```python
from build123d import *

# Parameters (mm, degrees)
F0_W      = 550
F0_H      = 875
F1_DEPTH  = 20
F2_W      = 510
F2_H      = 835
F3_DEPTH  = 20.001
F4_W      = 80
F4_H      = 3
F5_DEPTH  = 510
F6_W      = 20
F6_H      = 20
F7_DEPTH  = 400
F8_W      = 20
F8_H      = 20
F9_DEPTH  = 835
F10_W     = 20
F10_H     = 20
F11_DEPTH = 835
F12_W     = 20
F12_H     = 20
F13_DEPTH = 510
F15_W     = 3
F15_H     = 80
F16_DEPTH = 835
F17_W     = 3
F17_H     = 80
F18_DEPTH = 835
F19_W     = 20
F19_H     = 20
F20_DEPTH = 510
F14_W     = 80
F14_H     = 3
F14_W_2   = 3
F14_H_2   = 80
F21_DEPTH = 380
F22_DEPTH = 400
F23_W     = 20
F23_H     = 20
F24_DEPTH = 330
F25_W     = 20
F25_H     = 20
F26_DEPTH = 510
F27_W     = 20
F27_H     = 20
F28_DEPTH = 60
F29_W     = 20
F29_H     = 20
F30_DEPTH = 510
F31_W     = 20
F31_H     = 20
F32_DEPTH = 510
F33_W     = 20
F33_H     = 20
F34_DEPTH = 40
F35_W     = 20
F35_H     = 20
F36_DEPTH = 40
F37_W     = 20
F37_H     = 20
F38_DEPTH = 710
F40_DEPTH = 40


with BuildPart() as f1:
    # F0 (on Top) → F1 (new body)
    with BuildSketch(Plane.XY):
        with Locations((132.149377, 45.573115)):
            Rectangle(F0_W, F0_H)
    extrude(amount=F1_DEPTH)

    # F2 (on face) → F3 (cut, through all)
    with BuildSketch(Plane(origin=(0, 0, 0), x_dir=(1, 0, 0), z_dir=(0, 0, -1))):
        with Locations((132.149377, -45.573115)):
            Rectangle(F2_W, F2_H)
    extrude(amount=-F3_DEPTH, mode=Mode.SUBTRACT)

    # F4 (on face) → F5 (join, through all)
    with BuildSketch(Plane.YZ.offset(-122.850623)):
        with Locations((273.073115, 18.5)):
            Rectangle(F4_W, F4_H)
        with Locations((-221.926885, 18.5)):
            Rectangle(F4_W, F4_H)
    extrude(amount=F5_DEPTH)



with BuildPart() as f7:
    # F6 (on face) → F7 (new body)
    with BuildSketch(Plane.XY.offset(20)):
        with Locations((-132.850623, -381.926885)):
            Rectangle(F6_W, F6_H)
        with Locations((397.149377, -381.926885)):
            Rectangle(F6_W, F6_H)
        with Locations((-132.850623, 473.073115)):
            Rectangle(F6_W, F6_H)
        with Locations((397.149377, 473.073115)):
            Rectangle(F6_W, F6_H)
    extrude(amount=F7_DEPTH)

    # F8 (on face) → F9 (join, through all)
    with BuildSketch(Plane(origin=(0, -371.926885, 0), x_dir=(-1, 0, 0), z_dir=(0, 1, 0))):
        with Locations((-397.149377, 410)):
            Rectangle(F8_W, F8_H)
    extrude(amount=F9_DEPTH)

    # F10 (on face) → F11 (join, through all)
    with BuildSketch(Plane.XZ.offset(-463.073115)):
        with Locations((-132.850623, 410)):
            Rectangle(F10_W, F10_H)
    extrude(amount=F11_DEPTH)

    # F12 (on face) → F13 (join, through all)
    with BuildSketch(Plane(origin=(387.149377, 0, 0), x_dir=(0, -1, 0), z_dir=(-1, 0, 0))):
        with Locations((381.926885, 410)):
            Rectangle(F12_W, F12_H)
    extrude(amount=F13_DEPTH)

    # F15 (on face) → F16 (join, through all)
    with BuildSketch(Plane.XZ.offset(-463.073115)):
        with Locations((405.649377, 360)):
            Rectangle(F15_W, F15_H)
    extrude(amount=F16_DEPTH)

    # F17 (on face) → F18 (join, through all)
    with BuildSketch(Plane.XZ.offset(-463.073115)):
        with Locations((-141.350623, 360)):
            Rectangle(F17_W, F17_H)
    extrude(amount=F18_DEPTH)

    # F19 (on face) → F20 (join, through all)
    with BuildSketch(Plane(origin=(387.149377, 0, 0), x_dir=(0, -1, 0), z_dir=(-1, 0, 0))):
        with Locations((-473.073115, 410)):
            Rectangle(F19_W, F19_H)
    extrude(amount=F20_DEPTH)


with BuildPart() as f1_1:
    add(f1.part)

    add(f7.part)  # F21 merges F7
    # F14 (on face) → F21 (join, through all)
    with BuildSketch(Plane.XY.offset(20)):
        with Locations((132.149377, -373.426885)):
            Rectangle(F14_W, F14_H)
        with Locations((132.149377, 464.573115)):
            Rectangle(F14_W, F14_H)
        with Locations((388.649377, 273.073115)):
            Rectangle(F14_W_2, F14_H_2)
        with Locations((388.649377, -221.926885)):
            Rectangle(F14_W_2, F14_H_2)
        with Locations((-124.350623, -221.926885)):
            Rectangle(F14_W_2, F14_H_2)
        with Locations((-124.350623, 273.073115)):
            Rectangle(F14_W_2, F14_H_2)
    extrude(amount=F21_DEPTH)

    # F14 (on face) → F22 (join, through all)
    with BuildSketch(Plane.XY.offset(20)):
        with Locations((132.149377, -373.426885)):
            Rectangle(F14_W, F14_H)
        with Locations((132.149377, 464.573115)):
            Rectangle(F14_W, F14_H)
        with Locations((388.649377, 273.073115)):
            Rectangle(F14_W_2, F14_H_2)
        with Locations((388.649377, -221.926885)):
            Rectangle(F14_W_2, F14_H_2)
        with Locations((-124.350623, -221.926885)):
            Rectangle(F14_W_2, F14_H_2)
        with Locations((-124.350623, 273.073115)):
            Rectangle(F14_W_2, F14_H_2)
    extrude(amount=F22_DEPTH)

    # F23 (on face) → F24 (join)
    with BuildSketch(Plane.XY.offset(420)):
        with Locations((-132.850623, -381.926885)):
            Rectangle(F23_W, F23_H)
        with Locations((397.149377, -381.926885)):
            Rectangle(F23_W, F23_H)
    extrude(amount=F24_DEPTH)

    # F25 (on face) → F26 (join, through all)
    with BuildSketch(Plane(origin=(387.149377, 0, 0), x_dir=(0, -1, 0), z_dir=(-1, 0, 0))):
        with Locations((381.926885, 740)):
            Rectangle(F25_W, F25_H)
    extrude(amount=F26_DEPTH)

    # F27 (on face) → F28 (join)
    with BuildSketch(Plane.XZ.offset(391.926885)):
        with Locations((-132.850623, 10)):
            Rectangle(F27_W, F27_H)
        with Locations((397.149377, 10)):
            Rectangle(F27_W, F27_H)
        with Locations((-132.850623, 740)):
            Rectangle(F27_W, F27_H)
        with Locations((397.149377, 740)):
            Rectangle(F27_W, F27_H)
    extrude(amount=F28_DEPTH)

    # F29 (on face) → F30 (join, through all)
    with BuildSketch(Plane.YZ.offset(-122.850623)):
        with Locations((-441.926885, 740)):
            Rectangle(F29_W, F29_H)
    extrude(amount=F30_DEPTH)

    # F31 (on face) → F32 (join, through all)
    with BuildSketch(Plane(origin=(387.149377, 0, 0), x_dir=(0, -1, 0), z_dir=(-1, 0, 0))):
        with Locations((441.926885, 10)):
            Rectangle(F31_W, F31_H)
    extrude(amount=F32_DEPTH)

    # F33 (on face) → F34 (join)
    with BuildSketch(Plane(origin=(-142.850623, 0, 0), x_dir=(0, -1, 0), z_dir=(-1, 0, 0))):
        with Locations((441.926885, 10)):
            Rectangle(F33_W, F33_H)
        with Locations((441.926885, 740)):
            Rectangle(F33_W, F33_H)
    extrude(amount=F34_DEPTH)

    # F35 (on face) → F36 (join)
    with BuildSketch(Plane.YZ.offset(407.149377)):
        with Locations((-441.926885, 10)):
            Rectangle(F35_W, F35_H)
        with Locations((-441.926885, 740)):
            Rectangle(F35_W, F35_H)
    extrude(amount=F36_DEPTH)

    # F37 (on face) → F38 (join, through all)
    with BuildSketch(Plane(origin=(0, 0, 730), x_dir=(1, 0, 0), z_dir=(0, 0, -1))):
        with Locations((437.149377, 441.926885)):
            Rectangle(F37_W, F37_H)
        with Locations((-172.850623, 441.926885)):
            Rectangle(F37_W, F37_H)
    extrude(amount=F38_DEPTH)

    # F39 (on face) → F40 (join, through all)
    with BuildSketch(Plane.XZ.offset(391.926885)):
        Polygon((114.305049, 733), (-122.850623, 733), (-122.850623, 730), (114.305049, 730), (387.149377, 730), (387.149377, 733), align=None)
    extrude(amount=F40_DEPTH)


solid = f1_1.part
```
For this review, take the finished solid that the model builds, in its own axes (mm). A direction names the side the tool comes from. Give positions to 0.01 mm unless a question says otherwise; leave off trailing zeros. Order: outer loops, then holes, each group sorted by start corner. A loop starts at its lowest first (then second) coordinate and runs counter-clockwise, first axis right, second up.
1) Take a section at A-A (y = 218). Give the boundary of the cut face in (x, z).
2) For faces 1 (the face through (404.149, 51, 359)), 2 (the face through (129, -222, 17)), 3 (the face through (133, -371.927, 225)), list the 3-axis set-ups (+Z, -Z, +X, -X, +Y, -Y) from which the entire face can be reached by the end or side of a thin tool; tool diameter is ignored.
3) Wall thickness on line 1 (Y direction, x = 92.5, z = 83); line 2 (X direction, y = -381, z = 100); line 3 (Z direction, x = -123, y = -335.5): over which ranges is each line inside the solid? List them lowest first.
4) Insertion check: pin 1 (3 mm diameter, centred on x = 225, y = 284.5, fed in from -Z); pin 2 (3.5 mm diameter, centred on x = -124, z = 119.5, fed in from -Y); pin 3 (16 mm diameter, centred on y = 476.5, z = 174, fed in from +X). Each pin has a flat end and moves straight along its axis. Give the tip position at first contact, or say it passes through.
5) The part is to be moulded in two halves that separate along Y. For faces 4 (the face through (-176, -431.927, 370)), 5 (the face through (-125.851, 273, 207)), 6 (the face through (-142.851, -6, 345)), say which applies: released by +Y, released by -Y, zero draft, split by the parting line, or undercut.
6) Take a section at C-C (x = 111). State how many separate pieces and enclosed holes the cut face has, then the cut area to 3 significant figures.
7) Take a section at B-B (z = 567). Give the boundary of the cut face in (x, y), then the cut area to 3 significant figures.
Derived:
1. outline: (-142.85, 0) - (-122.85, 0) - (-122.85, 20) - (-142.85, 20) - close; (-142.85, 320) - (-139.85, 320) - (-139.85, 400) - (-122.85, 400) - (-122.85, 420) - (-142.85, 420) - close; (387.15, 0) - (407.15, 0) - (407.15, 20) - (387.15, 20) - close; (387.15, 400) - (404.15, 400) - (404.15, 320) - (407.15, 320) - (407.15, 420) - (387.15, 420) - close
2. face 1: none
2. face 2: -Z
2. face 3: +Z, -Z
3. line 1: y = -374.93 to -371.93, 463.07 to 466.07
3. line 2: x = -142.85 to -122.85, 387.15 to 407.15
3. line 3: z = 0 to 20, 400 to 420
4. pin 1: stops at z = 17
4. pin 2: stops at y = -391.93
4. pin 3: stops at x = 407.15
5. face 4: released by +Y
5. face 5: undercut
5. face 6: zero draft
6. separate pieces: 6
6. enclosed holes: 0
6. area: 5,680 mm2
7. outline: (-182.85, -451.93) - (-162.85, -451.93) - (-162.85, -431.93) - (-182.85, -431.93) - close; (-142.85, -391.93) - (-122.85, -391.93) - (-122.85, -371.93) - (-142.85, -371.93) - close; (387.15, -391.93) - (407.15, -391.93) - (407.15, -371.93) - (387.15, -371.93) - close; (427.15, -451.93) - (447.15, -451.93) - (447.15, -431.93) - (427.15, -431.93) - close
7. area: 1,600 mm2
